Autodesk Fusion 360 part; units mm, degrees
sketch "Skizze1" plane through (0, 0, 0) normal (1, 0, 0) x (0, 0, -1)
  line L0 (-75, 0) -> (90, 0)
  line L1 (-13, 0) -> (-13, 7.9)
  line L2 (-13, 7.9) -> (-9, 7.9)
  line L3 (-9, 7.9) -> (-9, 7)
  line L4 (-9, 7) -> (8, 7)
  line L5 (8, 7) -> (8, 8)
  line L6 (8, 8) -> (12, 8)
  line L7 (12, 8) -> (12, 0)
  dimension "d1" = 7.9
  dimension "d2" = 4
  dimension "d3" = 17
  dimension "d4" = 4
revolve "Drehen1" add sketch "Skizze1" angle 360 about axis through (0, 0, 75) along (0, 0, -1) makes body 1
hole "Bohrung1" at (0, 0, 13) direction (0, 0, -1) diameter 12.5 end through all bodies 1 1
ref_plane "Arbeitsebene2" through (0, 7, 0.9561) normal (0, 1, 0) x (-1, 0, 0)
sketch "Skizze3" plane through (0, 7, 0.9561) normal (0, 1, 0) x (1, 0, 0)
  point P0 (0, -6)
hole "Bohrung2" at (0, 7, 6.9561) direction (0, -1, 0) diameter 4 depth 14 tip angle 180 bodies 1
copy_body "Körper->Berechn1" bodies 1 removing the originals makes body 2 in component "gasChargingCryoarmGuide"
component "gasChargingCryoarmGuide" placed x (1, 0, 0) y (0, 1, 0) z (0, 0, 1) at (0, 0, 0)
equation "d1 = ( 15.8 / 2 ) * 1 mm"
The listing builds one solid part. Answer for the finished solid, in the listing's coordinates (mm). A direction names the side the tool comes from. Coordinates: 2 decimals unless noted, no trailing zeros. Loops run counter-clockwise (first coordinate to the right, second up) from the corner with the lowest first, then second, coordinate; pieces in that order, holes last. Notation, with made-up numbers: M 47,61 L 72,61 A33 cw 72,89 Z; hole C 48.25,89 d1. An arc over 180 degrees is marked long. Answer as CSV lines item,"result". Start each with the question number.
(1) Find the intervals of material crossed by L1, parallel to Y at x = 0, z = -1.5; L2, parallel to Z at x = 6.75, y = 2; L3, parallel to Z at x = 0, y = 6.4, in increasing order. Write a range as [from, to].
(2) The part is cut by section B-B (x = 3.25). Give the vertices of the cut face in (y, z), and give its area (3 significant figures).
(3) The part is cut by section D-D (z = 1.25). Give the vertices of the cut face in (x, y).
(4) The mould has two halves that part along Y. Classify faces 1 (the cylindrical face through (-1.88, -5.96, 0.32)), 2 (the flat face through (6.5, 0.5, 13)), 3 (the cylindrical face through (-4.807, -6.269, 10.972)): pulls with the +Y half, pulls with the -Y half, needs draft (parallel to the pull), parting line crosses it, or undercut.
(5) The part is cut by section C-C (x = 0). Give the vertices of the cut face in (y, z).
(6) For faces 4 (the flat face through (-4, -5, -12)), 5 (the flat face through (-6, 4, -8)), determine the directions among +Z, -Z, +X, -X, +Y, -Y from which every point of the face is accessible in a straight line to the end or side of a thin tool.
(7) The part is cut by section A-A (y = 0). Give the vertices of the cut face in (x, z).
(8) Given pin 1 (1.5 mm diameter, centred on x = -4.5, z = -0.5, fed in from -Y); pin 2 (4.5 mm diameter, centred on x = 0, z = 6.96, fed in from +Y); pin 3 (5 mm diameter, centred on x = -0.5, y = -3, fed in from +Z); pin 4 (4 mm diameter, centred on x = -5, z = -8.5, fed in from -Y), each flat-ended and moving along its own axis, determine where each tip first touches the part or whether it passes through.
Determined:
1,L1,"[-7, -6.25], [6.25, 7]"
1,L2,"[-12, -8], [9, 13]"
1,L3,"[-12, 4.96], [8.96, 13]"
2,outline,"M -7.31,-12 L -5.34,-12 L -5.34,13 L -7.2,13 L -7.2,9 L -6.2,9 L -6.2,-8 L -7.31,-8 Z; M 5.34,-12 L 7.31,-12 L 7.31,-8 L 6.2,-8 L 6.2,9 L 7.2,9 L 7.2,13 L 5.34,13 Z"
2,area,"60.0 mm2"
3,outline,"C 0,0 d14; hole C 0,0 d12.5"
4,face 1,"undercut"
4,face 2,"needs draft"
4,face 3,"parting line crosses it"
5,outline,"M -8,-12 L -6.25,-12 L -6.25,4.96 L -7,4.96 L -7,-8 L -8,-8 Z; M -7.9,9 L -7,9 L -7,8.96 L -6.25,8.96 L -6.25,13 L -7.9,13 Z; M 6.25,-12 L 8,-12 L 8,-8 L 7,-8 L 7,4.96 L 6.25,4.96 Z; M 6.25,8.96 L 7,8.96 L 7,9 L 7.9,9 L 7.9,13 L 6.25,13 Z"
6,face 4,"-Z, +X, -X, +Y, -Y"
6,face 5,"none"
7,outline,"M -8,-12 L -6.25,-12 L -6.25,13 L -7.9,13 L -7.9,9 L -7,9 L -7,-8 L -8,-8 Z; M 6.25,-12 L 8,-12 L 8,-8 L 7,-8 L 7,9 L 7.9,9 L 7.9,13 L 6.25,13 Z"
8,pin 1,"y = -5.91"
8,pin 2,"y = 7.9"
8,pin 3,"through"
8,pin 4,"y = -7.42"
